from build123d import *

# Parameters (mm, degrees)
FILLET_R     = 9
CHAMFER_SIZE = 1.1


with BuildPart() as part:
    # Sketch → Revolution (revolve)
    with BuildSketch(Plane.XZ):
        Polygon((4, 46), (4, 8), (2, 8), (2, 5), (5, 5), (5, 0), (17, 0), (17, 5), (7, 5), (7, 30), (5, 46), align=None)
    revolve(axis=Axis((0, 0, 0), (0, 0, 1)))

    # Fillet
    fillet_edges = [part.edges().sort_by_distance(p)[0] for p in [
        (-7, 0, 5),
    ]]
    fillet(fillet_edges, radius=FILLET_R)

    # Chamfer
    chamfer_edges = [part.edges().sort_by_distance(p)[0] for p in [
        (-17, 0, 5),
        (-17, 0, 0),
    ]]
    chamfer(chamfer_edges, length=CHAMFER_SIZE)


solid = part.part
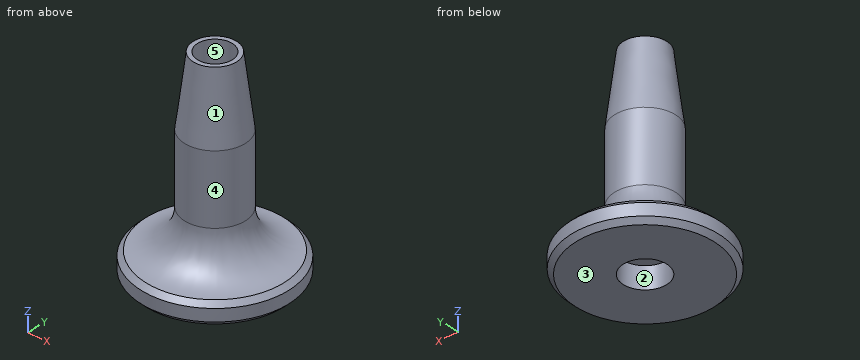
CAD build for the part. Positions are in the model's coordinates, mm. Face numbers are marked on the shaded views. A direction names the side the tool comes from. Round coordinates to 2 decimals unless told otherwise and drop trailing zeros. Order: outer loops, then holes, each group sorted by start corner. A loop starts at its lowest first (then second) coordinate and runs counter-clockwise, first axis right, second up. Notation, with made-up numbers: (15.5, 81.25) - (30.5, 81.25) arc R25 cw to (30.5, 112.25) - close; hole circle Ø10 at (35.25, -17.5). An arc over 180 degrees is marked (long way). Return JSON: item names as keys, results as strings.
(1) Cut at B-B (z = 38). Give the cut face in (x, y), then the cut area to 3 significant figures.
Answer key:
{"outline": "circle Ø12 at (0, 0); hole circle Ø8 at (0, 0)", "area": "62.8 mm^2"}
(2) Pull direction X, two halves, no side cores. Call the marked faces 3, 4 and 5: +X half, -X half, draft (parallel to the pull), parting line (faces both ways), or undercut.
Answer key:
{"face 3": "draft", "face 4": "parting line", "face 5": "undercut"}
(3) Wall check: probe 1 along Y at (x, z) = (1, 33); probe 2 along Y at (x, z) = (0, 5.9); probe 3 along Z at (x, y) = (3.5, -1). Give the ranges that are in metal, low to high. Write a range as from..to.
Answer key:
{"probe 1": "y = -6.55..-3.87, 3.87..6.55", "probe 2": "y = -12.08..-2, 2..12.08", "probe 3": "z = 5..8"}
(4) Tool access for the marked faces 1 and 2: list every direction of +Z, -Z, +X, -X, +Y, -Y with a clear straight run to the whole face (end or side of a thin tool).
Answer key:
{"face 1": "+Z", "face 2": "-Z"}
(5) Cut at A-A (z = 21). Give the cut face in (x, y).
Answer key:
{"outline": "circle Ø14 at (0, 0); hole circle Ø8 at (0, 0)"}
(6) Pin check, flat tips, straight feed: pin 1 Ø1 at (x, z) = (2, 9) entering from -Y; pin 2 Ø1 at (y, z) = (3.5, 32.5) entering from +X; pin 3 Ø2 at (x, y) = (10, 2.5) entering from +Z; pin 4 Ø3 at (x, y) = (0, 0) entering from -Z. Stop position of each tip, or through.
Answer key:
{"pin 1": "stops at y = -8.66", "pin 2": "stops at x = 5.99", "pin 3": "stops at z = 7.98", "pin 4": "passes through"}
